from build123d import *

# Parameters (mm, degrees)
SKETCH1_W           = 73.969271166
SKETCH1_H           = 49.312847444
BOSS_EXTRUDE1_DEPTH = 3.000000096
SKETCH2_W           = 31.971798189
SKETCH2_H           = 4.7152652
BOSS_EXTRUDE2_DEPTH = 6.35


with BuildPart() as part:
    # Sketch1 → Boss-Extrude1 (new body)
    with BuildSketch(Plane.XY):
        Rectangle(SKETCH1_W, SKETCH1_H)
    extrude(amount=BOSS_EXTRUDE1_DEPTH)

    # Sketch2 → Boss-Extrude2 (add)
    with BuildSketch(Plane.XY):
        with Locations((19.598546823, 22.298791122)):
            Rectangle(SKETCH2_W, SKETCH2_H)
    extrude(amount=-BOSS_EXTRUDE2_DEPTH)


solid = part.part
Can you work these out from the model? Positions are in its coordinate system, mm. A direction names the side the tool comes from. Give positions to 0.01 mm unless a question says otherwise; leave off trailing zeros. Loops run counter-clockwise (first coordinate to the right, second up) from the corner with the lowest first, then second, coordinate; pieces in that order, holes last. Notation, with made-up numbers: (39.5, -36.5) - (95.5, -36.5) arc R33 cw to (95.5, -3.5) - close; hole circle Ø9 at (-20, 79.25). An arc over 180 degrees is marked (long way). Return JSON: item names as keys, results as strings.
1. I'm going to push flat-ended pins straight in: pin 1 Ø4 at (x, y) = (25, -5) entering from -Z; pin 2 Ø1.9 at (x, z) = (22, -4) entering from -Y; pin 3 Ø2.5 at (y, z) = (23, -2) entering from +X. Where does each tip first touch, or does it pass through?
Output values:
{"pin 1": "stops at z = 0", "pin 2": "stops at y = 19.94", "pin 3": "stops at x = 35.58"}
2. I want a section at B-B on x = 20. Please give me the cut outline in (y, z), and give its area (3 significant figures).
Output values:
{"outline": "(-24.66, 0) - (19.94, 0) - (19.94, -6.35) - (24.66, -6.35) - (24.66, 3) - (-24.66, 3) - close", "area": "178 mm²"}
3. I want a section at D-D on y = -17. Please give me the cut outline in (x, z), and give its area (3 significant figures).
Output values:
{"outline": "(-36.98, 0) - (36.98, 0) - (36.98, 3) - (-36.98, 3) - close", "area": "222 mm²"}
4. I want a section at C-C on z = -1. Please give me the cut outline in (x, y), and give its area (3 significant figures).
Output values:
{"outline": "(3.61, 19.94) - (35.58, 19.94) - (35.58, 24.66) - (3.61, 24.66) - close", "area": "151 mm²"}
5. If I drill on line 1 (Z direction, x = 14, y = 2); line 2 (Y direction, x = 25.5, z = -3.5), over which ranges is the centre line in solid material (lowest first)?
Output values:
{"line 1": "z = 0 to 3", "line 2": "y = 19.94 to 24.66"}
6. I want a section at A-A on y = 21. Please give me the cut outline in (x, z).
Output values:
{"outline": "(-36.98, 0) - (3.61, 0) - (3.61, -6.35) - (35.58, -6.35) - (35.58, 0) - (36.98, 0) - (36.98, 3) - (-36.98, 3) - close"}
7. For faces 1 (the face through (3.613, 22, -3)), 2 (the face through (19, 19.941, -3)), 3 (the face through (35.584, 22, -3)), which set-ups out of +Z, -Z, +X, -X, +Y, -Y let a thin tool reach every point of the face, with its end or its side?
Output values:
{"face 1": "-Z, -X, +Y, -Y", "face 2": "-Z, +X, -X, -Y", "face 3": "-Z, +X, +Y, -Y"}
